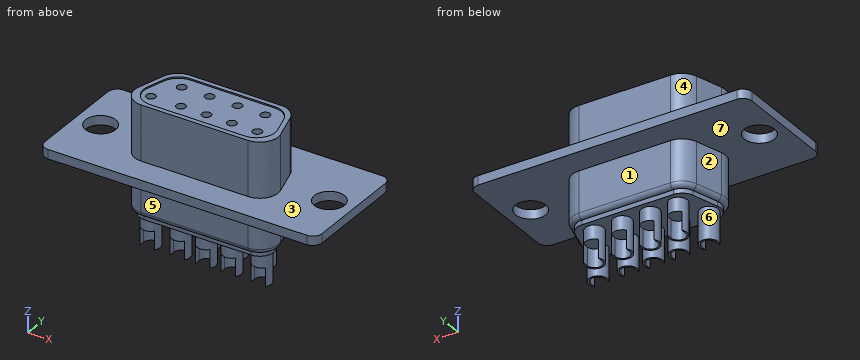
from build123d import *

# Parameters (mm, degrees)
SKETCH1_W       = 30.3
SKETCH1_H       = 12.7
EXTRUDE1_DEPTH  = 1
SKETCH2_R       = 1.65
EXTRUDE2_DEPTH  = 17.45736917
EXTRUDE3_DEPTH  = 6
FILLET2_R       = 1
EXTRUDE4_DEPTH  = 5
FILLET1_R       = 2
FILLET3_R       = 0.5
EXTRUDE5_DEPTH  = 0.5
SKETCH6_R       = 1
EXTRUDE6_DEPTH  = 3.5
EXTRUDE15_DEPTH = 2
EXTRUDE16_START = 5.85
SKETCH8_R       = 0.5
SKETCH8_R_2     = 0.502640461
EXTRUDE16_DEPTH = 5.85


with BuildPart() as part:
    # Sketch1 → Extrude1 (new body)
    with BuildSketch(Plane.XY):
        Rectangle(SKETCH1_W, SKETCH1_H)
    extrude(amount=EXTRUDE1_DEPTH)

    # Sketch2 → Extrude2 (cut, through all)
    with BuildSketch(Plane.XY.offset(1)):
        with Locations((-12.5, 0)):
            Circle(SKETCH2_R)
        with Locations((12.5, 0)):
            Circle(SKETCH2_R)
    extrude(amount=-EXTRUDE2_DEPTH, mode=Mode.SUBTRACT)

    # Sketch3 → Extrude3 (add)
    with BuildSketch(Plane.XY.offset(1)):
        Polygon((-6.5, 3.45), (6.5, 3.45), (8.5, -3.45), (-8.5, -3.45), align=None)
        Polygon((-6.1243471, 2.95), (6.1243471, 2.95), (7.834492027, -2.95), (-7.834492027, -2.95), align=None, mode=Mode.SUBTRACT)
    extrude(amount=EXTRUDE3_DEPTH)

    # Fillet2
    fillet2_edges = [part.edges().sort_by_distance(p)[0] for p in [
        (15.15, -6.35, 0.5),
        (-15.15, -6.35, 0.5),
        (-15.15, 6.35, 0.5),
        (15.15, 6.35, 0.5),
    ]]
    fillet(fillet2_edges, radius=FILLET2_R)

    # Sketch4 → Extrude4 (add)
    with BuildSketch(Plane(origin=(0, 0, 0), x_dir=(-1, 0, 0), z_dir=(0, 0, -1))):
        Polygon((-6.5, 3.45), (-8.5, -3.45), (8.5, -3.45), (6.5, 3.45), align=None)
    extrude(amount=EXTRUDE4_DEPTH)

    # Fillet1
    fillet1_edges = [part.edges().sort_by_distance(p)[0] for p in [
        (8.5, -3.45, 4),
        (6.5, 3.45, 4),
        (-6.5, 3.45, 4),
        (-7.834492027, -2.95, 4),
        (-6.1243471, 2.95, 4),
        (6.1243471, 2.95, 4),
        (7.834492027, -2.95, 4),
        (-8.5, -3.45, 4),
        (-6.5, 3.45, -2.5),
        (6.5, 3.45, -2.5),
        (8.5, -3.45, -2.5),
        (-8.5, -3.45, -2.5),
    ]]
    fillet(fillet1_edges, radius=FILLET1_R)

    # Fillet3
    fillet3_edges = [part.edges().sort_by_distance(p)[0] for p in [
        (-7.338610987, 0.556792096, -5),
        (0, -3.45, -5),
        (0, 3.45, -5),
        (7.338610987, 0.556792096, -5),
        (6.198724282, 3.048997216, -5),
        (7.436965325, -2.651335883, -5),
        (-6.198724282, 3.048997216, -5),
        (-7.436965325, -2.651335883, -5),
    ]]
    fillet(fillet3_edges, radius=FILLET3_R)

    # Sketch5 → Extrude5 (add)
    with BuildSketch(Plane(origin=(0, 0, -5), x_dir=(-1, 0, 0), z_dir=(0, 0, -1))):
        with BuildLine():
            Line((-4.997388399, 2.95), (4.997388399, 2.95))
            ThreePointArc((4.997388399, 2.95), (5.898390312, 2.649247912), (6.438087948, 1.867594072))
            Line((6.438087948, 1.867594072), (7.278667659, -1.032405928))
            ThreePointArc((7.278667659, -1.032405928), (7.037216021, -2.351001912), (5.837968109, -2.95))
            Line((5.837968109, -2.95), (-5.837968109, -2.95))
            ThreePointArc((-5.837968109, -2.95), (-7.037216021, -2.351001912), (-7.278667659, -1.032405928))
            Line((-7.278667659, -1.032405928), (-6.438087948, 1.867594072))
            ThreePointArc((-6.438087948, 1.867594072), (-5.898390312, 2.649247912), (-4.997388399, 2.95))
        make_face()
    extrude(amount=EXTRUDE5_DEPTH)

    # Sketch6 → Extrude6 (add)
    with BuildSketch(Plane(origin=(0, 0, -5.5), x_dir=(-1, 0, 0), z_dir=(0, 0, -1))):
        with Locations((-4.570282288, 1.45)):
            Circle(SKETCH6_R)
        with Locations((-1.523427429, 1.45)):
            Circle(SKETCH6_R)
        with Locations((1.523427429, 1.45)):
            Circle(SKETCH6_R)
        with Locations((4.570282288, 1.45)):
            Circle(SKETCH6_R)
        with Locations((6.067542907, -1.45)):
            Circle(SKETCH6_R)
        with Locations((2.783771454, -1.45)):
            Circle(SKETCH6_R)
        with Locations((0, -1.45)):
            Circle(SKETCH6_R)
        with Locations((-2.783771454, -1.45)):
            Circle(SKETCH6_R)
        with Locations((-6.067542907, -1.45)):
            Circle(SKETCH6_R)
    extrude(amount=EXTRUDE6_DEPTH)

    # Sketch7 → Extrude15 (cut)
    with BuildSketch(Plane(origin=(0, 0, -9), x_dir=(-1, 0, 0), z_dir=(0, 0, -1))):
        with BuildLine():
            Line((-2.323427429, 1.45), (-2.323427429, 2.45))
            Line((-2.323427429, 2.45), (-0.723427429, 2.45))
            Line((-0.723427429, 2.45), (-0.723427429, 1.45))
            ThreePointArc((-0.723427429, 1.45), (-1.523427429, 0.65), (-2.323427429, 1.45))
        make_face()
        with BuildLine():
            Line((-5.370282288, 1.45), (-5.370282288, 2.45))
            Line((-5.370282288, 2.45), (-3.770282288, 2.45))
            Line((-3.770282288, 2.45), (-3.770282288, 1.45))
            ThreePointArc((-3.770282288, 1.45), (-4.570282288, 0.65), (-5.370282288, 1.45))
        make_face()
        with BuildLine():
            Line((-6.867542907, -1.45), (-6.867542907, -2.45))
            Line((-6.867542907, -2.45), (-5.267542907, -2.45))
            Line((-5.267542907, -2.45), (-5.267542907, -1.45))
            ThreePointArc((-5.267542907, -1.45), (-6.067542907, -0.65), (-6.867542907, -1.45))
        make_face()
        with BuildLine():
            Line((0.723427429, 1.45), (0.723427429, 2.45))
            Line((0.723427429, 2.45), (2.323427429, 2.45))
            Line((2.323427429, 2.45), (2.323427429, 1.45))
            ThreePointArc((2.323427429, 1.45), (1.523427429, 0.65), (0.723427429, 1.45))
        make_face()
        with BuildLine():
            Line((3.770282288, 1.45), (3.770282288, 2.45))
            Line((3.770282288, 2.45), (5.370282288, 2.45))
            Line((5.370282288, 2.45), (5.370282288, 1.45))
            ThreePointArc((5.370282288, 1.45), (4.570282288, 0.65), (3.770282288, 1.45))
        make_face()
        with BuildLine():
            Line((-1.983771454, -1.45), (-1.983771454, -2.45))
            Line((-1.983771454, -2.45), (-3.583771454, -2.45))
            Line((-3.583771454, -2.45), (-3.583771454, -1.45))
            ThreePointArc((-3.583771454, -1.45), (-2.783771454, -0.65), (-1.983771454, -1.45))
        make_face()
        with BuildLine():
            Line((0.8, -1.45), (0.8, -2.45))
            Line((0.8, -2.45), (-0.8, -2.45))
            Line((-0.8, -2.45), (-0.8, -1.45))
            ThreePointArc((-0.8, -1.45), (0, -0.65), (0.8, -1.45))
        make_face()
        with BuildLine():
            Line((3.583771454, -1.45), (3.583771454, -2.45))
            Line((3.583771454, -2.45), (1.983771454, -2.45))
            Line((1.983771454, -2.45), (1.983771454, -1.45))
            ThreePointArc((1.983771454, -1.45), (2.783771454, -0.65), (3.583771454, -1.45))
        make_face()
        with BuildLine():
            Line((6.867542907, -1.45), (6.867542907, -2.45))
            Line((6.867542907, -2.45), (5.267542907, -2.45))
            Line((5.267542907, -2.45), (5.267542907, -1.45))
            ThreePointArc((5.267542907, -1.45), (6.067542907, -0.65), (6.867542907, -1.45))
        make_face()
    extrude(amount=-EXTRUDE15_DEPTH, mode=Mode.SUBTRACT)

    # Sketch8 → Extrude16 (add)
    with BuildSketch(Plane.XY.offset(1).offset(EXTRUDE16_START)):
        with BuildLine():
            Line((-4.621735499, 2.95), (4.621735499, 2.95))
            ThreePointArc((4.621735499, 2.95), (5.823071382, 2.548997216), (6.542668231, 1.506792096))
            Line((6.542668231, 1.506792096), (7.093392869, -0.393207904))
            ThreePointArc((7.093392869, -0.393207904), (6.771457353, -2.151335883), (5.172460137, -2.95))
            Line((5.172460137, -2.95), (-5.172460137, -2.95))
            ThreePointArc((-5.172460137, -2.95), (-6.771457353, -2.151335883), (-7.093392869, -0.393207904))
            Line((-7.093392869, -0.393207904), (-6.542668231, 1.506792096))
            ThreePointArc((-6.542668231, 1.506792096), (-5.823071382, 2.548997216), (-4.621735499, 2.95))
        make_face()
        with Locations((-4.570282288, 1.45)):
            Circle(SKETCH8_R, mode=Mode.SUBTRACT)
        with Locations((-1.523427429, 1.45)):
            Circle(SKETCH8_R, mode=Mode.SUBTRACT)
        with Locations((1.523427429, 1.45)):
            Circle(SKETCH8_R, mode=Mode.SUBTRACT)
        with Locations((4.570282288, 1.45)):
            Circle(SKETCH8_R_2, mode=Mode.SUBTRACT)
        with Locations((5.567542907, -1.45)):
            Circle(SKETCH8_R, mode=Mode.SUBTRACT)
        with Locations((2.783771454, -1.45)):
            Circle(SKETCH8_R, mode=Mode.SUBTRACT)
        with Locations((0, -1.45)):
            Circle(SKETCH8_R, mode=Mode.SUBTRACT)
        with Locations((-2.783771454, -1.45)):
            Circle(SKETCH8_R, mode=Mode.SUBTRACT)
        with Locations((-6.067542907, -1.45)):
            Circle(SKETCH8_R, mode=Mode.SUBTRACT)
    extrude(amount=-EXTRUDE16_DEPTH)


solid = part.part
Can you work these out from the model? Positions are in its coordinate system, mm. Face numbers are marked on the shaded views. A direction names the side the tool comes from. Coordinates: 2 decimals unless noted, no trailing zeros. Write each loop counter-clockwise with the first axis right and the second up, starting at its lowest first coordinate (ties: lowest second). Pieces come first, ordered by that corner, then holes. Notation, with made-up numbers: (33.25, 50) - (41.25, 50) arc R30 ccw to (41.25, 87) - close; hole circle Ø6 at (31.25, 77). An arc over 180 degrees is marked (long way). Return JSON: item names as keys, results as strings. Group by question number.
Item 1: We'd pull the mould along Y, two halves only. Please class the marked faces 5, 6 and 7: pulls with the +Y half, pulls with the -Y half, needs draft (parallel to the pull), parting line crosses it, or undercut.
Item 2: If we section it at D-D (z = -2.5): Write out the boundary of the cut face in (x, y), then the cut area to 3 significant figures.
Item 3: If we section it at B-B (z = 3.5): Count the separate pieces of the cut face and the enclosed holes in it, then the cut area to 3 significant figures.
Item 4: Please list where these lines run through material, in increasing order: probe 1 along Y at (x, z) = (12.5, 0.7); probe 2 along Z at (x, y) = (2.5, -5.25); probe 3 along Y at (x, z) = (-1.5, -2.75).
Item 5: Which directions (+Z, -Z, +X, -X, +Y, -Y) give clear straight access to the entire face, cutting with the end or side of a thin tool? Please do the marked faces 1, 2, 3 and 4.
Item 6: If we section it at A-A (x = -12.5): Write out the boundary of the cut face in (y, z), then the cut area to 3 significant figures.
Item 7: I'm going to push flat-ended pins straight in: pin 1 Ø2 at (x, y) = (8, 3.5) entering from -Z; pin 2 Ø6 at (y, z) = (-3, -5) entering from +X; pin 3 Ø1.3 at (x, y) = (-4.5, 1.5) entering from -Z; pin 4 Ø2 at (y, z) = (-4, -6) entering from +X (3 decimals). Where does each tip first touch, or does it pass through?
Return value:
{
 "1": {"face 5": "pulls with the -Y half", "face 6": "undercut", "face 7": "needs draft"},
 "2": {"outline": "(-7.76, -0.89) arc R2 ccw to (-5.84, -3.45) - (5.84, -3.45) arc R2 ccw to (7.76, -0.89) - (6.92, 2.01) arc R2 ccw to (5, 3.45) - (-5, 3.45) arc R2 ccw to (-6.92, 2.01) - close", "area": "99.4 mm^2"},
 "3": {"separate pieces": "1", "enclosed holes": "9", "area": "92.3 mm^2"},
 "4": {"probe 1": "y = -6.35 to -1.65, 1.65 to 6.35", "probe 2": "z = 0 to 1", "probe 3": "y = -3.45 to 3.45"},
 "5": {"face 1": "-Z, +X, -X, +Y", "face 2": "-Z, -X, +Y", "face 3": "+Z", "face 4": "+Z, -X, +Y"},
 "6": {"outline": "(-6.35, 0) - (-1.65, 0) - (-1.65, 1) - (-6.35, 1) - close; (1.65, 0) - (6.35, 0) - (6.35, 1) - (1.65, 1) - close", "area": "9.40 mm^2"},
 "7": {"pin 1": "stops at z = 0", "pin 2": "stops at x = 7.84", "pin 3": "stops at z = -7", "pin 4": "passes through"}
}
